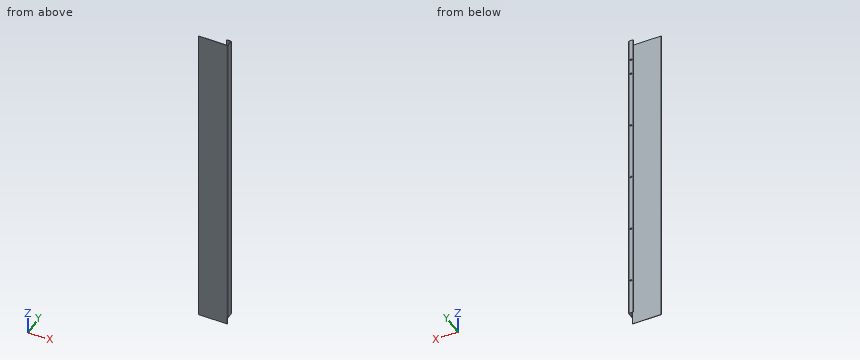
```python
from build123d import *

# Parameters (mm, degrees)
SKETCH1_W                    = 82
SKETCH1_H                    = 905.2
BASE_FLANGE1_DEPTH           = 1
EDGE_FLANGE1_STRIP_W         = 6
EDGE_FLANGE1_STRIP_H         = 1
EDGE_FLANGE1_STRIP_CUT_DEPTH = 905.2
EDGE_FLANGE1_DEPTH           = 905.2
EDGE_FLANGE2_STRIP_W         = 6
EDGE_FLANGE2_STRIP_H         = 1
EDGE_FLANGE2_STRIP_CUT_DEPTH = 905.2
EDGE_FLANGE2_DEPTH           = 905.2
SKETCH19_R                   = 2.5
CUT_EXTRUDE2_DEPTH           = 10
CUT_EXTRUDE3_START           = -905.2
CUT_EXTRUDE3_DEPTH           = 20.5


# Read off the part's stored shape, not the designer's step: Cut-Extrude3
# Sheet-metal steps are written as plain solids
with BuildPart() as part:
    # Sketch1 → Base-Flange1 (new body)
    with BuildSketch(Plane(origin=(0, 0, 0), x_dir=(1, 0, 0), z_dir=(0, 1, 0))):
        with Locations((41, 452.6)):
            Rectangle(SKETCH1_W, SKETCH1_H)
    extrude(amount=-BASE_FLANGE1_DEPTH)

    # Edge-Flange1 strip (across the edge) → Edge-Flange1 strip cut (cut)
    with BuildSketch(Plane(origin=(82, 0, 0), x_dir=(-1, 0, 0), z_dir=(0, 0, -1))):
        with Locations((-1, -0.5)):
            Rectangle(EDGE_FLANGE1_STRIP_W, EDGE_FLANGE1_STRIP_H)
    extrude(amount=EDGE_FLANGE1_STRIP_CUT_DEPTH, mode=Mode.SUBTRACT)

    # Edge-Flange1 section (across the edge) → Edge-Flange1 (add)
    with BuildSketch(Plane(origin=(82, 0, 0), x_dir=(-1, 0, 0), z_dir=(0, 0, -1))):
        with BuildLine():
            Line((0, 1), (0, 19))
            Line((0, 19), (1, 19))
            Line((1, 19), (1, 1))
            ThreePointArc((1, 1), (1.292893219, 0.292893219), (2, 0))
            Line((2, 0), (2, -1))
            ThreePointArc((2, -1), (0.585786438, -0.414213562), (0, 1))
        make_face()
    extrude(amount=EDGE_FLANGE1_DEPTH)

    # Edge-Flange2 strip (across the edge) → Edge-Flange2 strip cut (cut)
    with BuildSketch(Plane(origin=(81, 19, 0), x_dir=(0, -1, 0), z_dir=(0, 0, -1))):
        with Locations((-1, -0.5)):
            Rectangle(EDGE_FLANGE2_STRIP_W, EDGE_FLANGE2_STRIP_H)
    extrude(amount=EDGE_FLANGE2_STRIP_CUT_DEPTH, mode=Mode.SUBTRACT)

    # Edge-Flange2 section (across the edge) → Edge-Flange2 (add)
    with BuildSketch(Plane(origin=(81, 19, 0), x_dir=(0, -1, 0), z_dir=(0, 0, -1))):
        with BuildLine():
            Line((0, 1), (0, 12))
            Line((0, 12), (1, 12))
            Line((1, 12), (1, 1))
            ThreePointArc((1, 1), (1.292893219, 0.292893219), (2, 0))
            Line((2, 0), (2, -1))
            ThreePointArc((2, -1), (0.585786438, -0.414213562), (0, 1))
        make_face()
    extrude(amount=EDGE_FLANGE2_DEPTH)

    # Sketch19 → Cut-Extrude2 (cut)
    with BuildSketch(Plane(origin=(0, 19, 0), x_dir=(1, 0, 0), z_dir=(0, 1, 0))):
        with Locations(Location((75, 63, 0), (0, 0, 180))):
            Circle(SKETCH19_R)
        with Locations(Location((75, 108, 0), (0, 0, 180))):
            Circle(SKETCH19_R)
        with Locations(Location((75, 276, 0), (0, 0, 180))):
            Circle(SKETCH19_R)
        with Locations(Location((75, 444, 0), (0, 0, 180))):
            Circle(SKETCH19_R)
        with Locations(Location((75, 612, 0), (0, 0, 180))):
            Circle(SKETCH19_R)
        with Locations(Location((75, 780, 0), (0, 0, 180))):
            Circle(SKETCH19_R)
    extrude(amount=-CUT_EXTRUDE2_DEPTH, mode=Mode.SUBTRACT)

    # Cut-Extrude3 outline → Cut-Extrude3 (cut)
    with BuildSketch(Plane.XY.offset(CUT_EXTRUDE3_START)):
        with BuildLine():
            ThreePointArc((81, 1), (80.707106781, 0.292893219), (80, 0))
            Line((80, 0), (80, -1))
            ThreePointArc((80, -1), (81.414213562, -0.414213562), (82, 1))
            Line((82, 1), (82, 17))
            ThreePointArc((82, 17), (81.414213562, 18.414213562), (80, 19))
            Line((80, 19), (69, 19))
            Line((69, 19), (69, 18))
            Line((69, 18), (80, 18))
            ThreePointArc((80, 18), (80.707106781, 17.707106781), (81, 17))
            Line((81, 17), (81, 1))
        make_face()
    extrude(amount=CUT_EXTRUDE3_DEPTH, mode=Mode.SUBTRACT)


solid = part.part
```
Input: part model. Units: mm. Frame: model coordinates. Coordinates: 2 decimals unless noted, no trailing zeros. Write each loop counter-clockwise with the first axis right and the second up, starting at its lowest first coordinate (ties: lowest second). Pieces come first, ordered by that corner, then holes. Notation, with made-up numbers: (-18.75, 26) - (29.25, 26) arc R23 cw to (29.25, 45) - close; hole circle Ø2 at (35.25, 79). An arc over 180 degrees is marked (long way). Put each result on its own line as item: value. Start each with the question number.
1) Contact query for flat-ended pins moving along their axis: pin 1 (1.5 mm diameter, centred on y = 6.5, z = -654.5, fed in from -X); pin 2 (3 mm diameter, centred on x = 75, z = -63, fed in from +Y); pin 3 (0.5 mm diameter, centred on y = -0.5, z = -896, fed in from +X). Output: stop coordinate, or through.
2) Cut plane B-B (x = 11). Return the cut outline in (y, z), plus the area to 3 significant figures.
3) Cut plane A-A (z = -766.5). Return the cut outline in (x, y).
4) Ray query, L1, parallel to Y at x = 47, z = -316; L2, parallel to X at y = 11.5, z = -483.5; L3, parallel to X at y = 18.5, z = -780. Return the intervals inside material, ascending.
5) Cut plane C-C (y = 7.25). Return the cut outline in (x, z).
Resolved:
1. pin 1: stops at x = 81
1. pin 2: stops at y = 0
1. pin 3: stops at x = 80
2. outline: (-1, -905.2) - (0, -905.2) - (0, 0) - (-1, 0) - close
2. area: 905 mm2
3. outline: (0, -1) - (80, -1) arc R2 ccw to (82, 1) - (82, 17) arc R2 ccw to (80, 19) - (69, 19) - (69, 18) - (80, 18) arc R1 cw to (81, 17) - (81, 1) arc R1 cw to (80, 0) - (0, 0) - close
4. L1: y = -1 to 0
4. L2: x = 81 to 82
4. L3: x = 69 to 72.5, 77.5 to 81.32
5. outline: (81, -884.7) - (82, -884.7) - (82, 0) - (81, 0) - close
